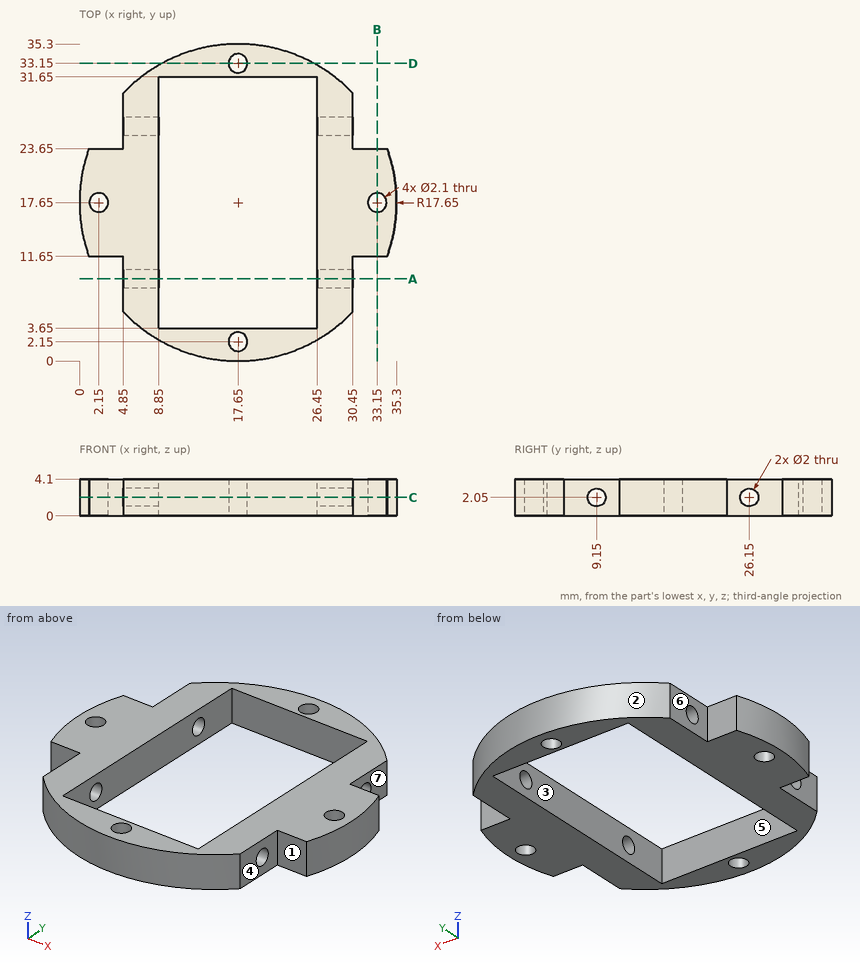
Here's the drawing with two shaded views (mm, measured from the low corner). I have some questions. A direction names the side the tool comes from. Round coordinates to 2 decimals unless told otherwise and drop trailing zeros. Loops run counter-clockwise (first coordinate to the right, second up) from the corner with the lowest first, then second, coordinate; pieces in that order, holes last.
Item 1: Will these pins go through, and if not, where does the flat tip stop? pin 1 Ø1.1 at (x, z) = (32, 3) entering from -Y; pin 2 Ø2 at (x, z) = (10.5, 1.5) entering from -Y; pin 3 Ø2 at (x, z) = (14, 2) entering from -Y.
Item 2: Suppose I cut it at A-A, the plane y = 9.15. Write out the boundary of the cut face in (x, z).
Item 3: Which directions (+Z, -Z, +X, -X, +Y, -Y) give clear straight access to the entire face, cutting with the end or side of a thin tool? Please do the marked faces 5, 6 and 7.
Item 4: Suppose I cut it at C-C, the plane z = 2.05. State how many separate pieces and enclosed holes the cut face has, then the cut area to 3 significant figures.
Item 5: Please list where these lines run through material, in increasing order: L1, parallel to X at y = 17.5, z = 3.9; L2, parallel to Y at x = 17.65, z = 2; L3, parallel to Y at x = 2.15, z = 1.
Item 6: Suppose I cut it at B-B, the plane x = 33.15. Write out the boundary of the cut face in (y, z), then the cut area to 3 significant figures.
Item 7: Suppose I cut it at D-D, the plane y = 33.15. Write out the boundary of the cut face in (x, z), then the cut area to 3 significant figures.
Item 8: If we mould it in two halves opening along Y, with no side actions, what happens to the marked faces 1, 2, 3 and 4? For each: +Y half, -Y half, draft (parallel to the pull), parting line (faces both ways), or undercut.
Reported:
1. pin 1: stops at y = 11.65
1. pin 2: stops at y = 1.11
1. pin 3: stops at y = 0.2
2. outline: (4.85, 0) - (8.85, 0) - (8.85, 1.05) - (4.85, 1.05) - close; (4.85, 3.05) - (8.85, 3.05) - (8.85, 4.1) - (4.85, 4.1) - close; (26.45, 0) - (30.45, 0) - (30.45, 1.05) - (26.45, 1.05) - close; (26.45, 3.05) - (30.45, 3.05) - (30.45, 4.1) - (26.45, 4.1) - close
3. face 5: +Z, -Z
3. face 6: +Z, -Z, -X, +Y
3. face 7: +Z, -Z, +X, +Y
4. separate pieces: 4
4. enclosed holes: 4
4. area: 386 mm2
5. L1: x = 0 to 1.11, 3.19 to 8.85, 26.45 to 32.11, 34.19 to 35.3
5. L2: y = 0 to 1.1, 3.2 to 3.65, 31.65 to 32.1, 34.2 to 35.3
5. L3: y = 11.65 to 16.6, 18.7 to 23.65
6. outline: (11.65, 0) - (16.6, 0) - (16.6, 4.1) - (11.65, 4.1) - close; (18.7, 0) - (23.65, 0) - (23.65, 4.1) - (18.7, 4.1) - close
6. area: 40.6 mm2
7. outline: (9.21, 0) - (16.6, 0) - (16.6, 4.1) - (9.21, 4.1) - close; (18.7, 0) - (26.09, 0) - (26.09, 4.1) - (18.7, 4.1) - close
7. area: 60.6 mm2
8. face 1: -Y half
8. face 2: +Y half
8. face 3: undercut
8. face 4: draft
